Check sheet for the modelled part. Datum: model origin and axes. Units: mm. A direction names the side the tool comes from. Give positions to 0.01 mm unless a question says otherwise; leave off trailing zeros. Loops run counter-clockwise (first coordinate to the right, second up) from the corner with the lowest first, then second, coordinate; pieces in that order, holes last. Notation, with made-up numbers: M 51,-37.75 L 105,-37.75 A25 cw 105,-16.75 Z; hole C 46,58 d8. An arc over 180 degrees is marked long. Put each result on its own line as item: value. Start each with the question number.
```python
from build123d import *

# Parameters (mm, degrees)
BOSS_EXTRUDE1_DEPTH = 3.175
CUT_EXTRUDE1_DEPTH  = 252.960239461
BOSS_EXTRUDE2_DEPTH = 3.175
SKETCH4_R           = 2.159
CUT_EXTRUDE2_DEPTH  = 252.960239461
SKETCH6_W           = 254
SKETCH6_H           = 106.880400145
CUT_EXTRUDE3_DEPTH  = 252.960239461


with BuildPart() as part:
    # Sketch1 → Boss-Extrude1 (new body)
    with BuildSketch(Plane(origin=(0, 0, 0), x_dir=(1, 0, 0), z_dir=(0, 1, 0))):
        Polygon((-152.4, 119.059630377), (-116.478975516, 154.980654861), (116.478975516, 154.980654861), (152.4, 119.059630377), (152.4, -164.698320655), (116.478975516, -200.619345139), (-116.478975516, -200.619345139), (-152.4, -164.698320655), align=None)
    extrude(amount=BOSS_EXTRUDE1_DEPTH)

    # Sketch2 → Cut-Extrude1 (cut, through all)
    with BuildSketch(Plane(origin=(0, 3.175, 0), x_dir=(1, 0, 0), z_dir=(0, 1, 0))):
        Polygon((-91.078975516, 129.580654861), (91.078975516, 129.580654861), (127, 93.659630377), (127, 8.930654861), (82.442975516, 8.930654861), (-74.314975516, 8.930654861), (-127, 8.930654861), (-127, 93.659630377), align=None)
        Polygon((127, -139.298320655), (91.078975516, -175.219345139), (-91.078975516, -175.219345139), (-127, -139.298320655), (-127, -54.569345139), (-74.314975516, -54.569345139), (82.442975516, -54.569345139), (127, -54.569345139), align=None)
    extrude(amount=-CUT_EXTRUDE1_DEPTH, mode=Mode.SUBTRACT)

    # Sketch5 → Boss-Extrude2 (add)
    with BuildSketch(Plane(origin=(0, 3.175, 0), x_dir=(1, 0, 0), z_dir=(0, 1, 0))):
        with BuildLine():
            Line((-116.478975516, 83.138605892), (-80.557951031, 119.059630377))
            ThreePointArc((-80.557951031, 119.059630377), (-78.800891411, 126.352814743), (-72.028975516, 129.580654861))
            Line((-72.028975516, 129.580654861), (-59.328975516, 129.580654861))
            Line((-59.328975516, 129.580654861), (-59.328975516, 154.980654861))
            Line((-59.328975516, 154.980654861), (-116.478975516, 154.980654861))
            Line((-116.478975516, 154.980654861), (-152.4, 119.059630377))
            Line((-152.4, 119.059630377), (-152.4, 65.258187686))
            Line((-152.4, 65.258187686), (-127, 65.258187686))
            Line((-127, 65.258187686), (-127, 77.958187686))
            ThreePointArc((-127, 77.958187686), (-123.351279088, 83.821819005), (-116.478975516, 83.138605892))
        make_face()
        with BuildLine():
            Line((127, 65.258187686), (127, 77.958187686))
            ThreePointArc((127, 77.958187686), (123.351279088, 83.821819005), (116.478975516, 83.138605892))
            Line((116.478975516, 83.138605892), (80.557951031, 119.059630377))
            ThreePointArc((80.557951031, 119.059630377), (78.800891411, 126.352814743), (72.028975516, 129.580654861))
            Line((72.028975516, 129.580654861), (59.328975516, 129.580654861))
            Line((59.328975516, 129.580654861), (59.328975516, 154.980654861))
            Line((59.328975516, 154.980654861), (116.478975516, 154.980654861))
            Line((116.478975516, 154.980654861), (152.4, 119.059630377))
            Line((152.4, 119.059630377), (152.4, 65.258187686))
            Line((152.4, 65.258187686), (127, 65.258187686))
        make_face()
        with BuildLine():
            Line((116.478975516, -128.777296171), (80.557951031, -164.698320655))
            ThreePointArc((80.557951031, -164.698320655), (78.800891411, -171.991505021), (72.028975516, -175.219345139))
            Line((72.028975516, -175.219345139), (59.328975516, -175.219345139))
            Line((59.328975516, -175.219345139), (59.328975516, -200.619345139))
            Line((59.328975516, -200.619345139), (116.478975516, -200.619345139))
            Line((116.478975516, -200.619345139), (152.4, -164.698320655))
            Line((152.4, -164.698320655), (152.4, -110.896877964))
            Line((152.4, -110.896877964), (127, -110.896877964))
            Line((127, -110.896877964), (127, -123.596877964))
            ThreePointArc((127, -123.596877964), (123.351279088, -129.460509283), (116.478975516, -128.777296171))
        make_face()
        with BuildLine():
            Line((-127, -110.896877964), (-127, -123.596877964))
            ThreePointArc((-127, -123.596877964), (-123.351279088, -129.460509283), (-116.478975516, -128.777296171))
            Line((-116.478975516, -128.777296171), (-80.557951031, -164.698320655))
            ThreePointArc((-80.557951031, -164.698320655), (-78.800891411, -171.991505021), (-72.028975516, -175.219345139))
            Line((-72.028975516, -175.219345139), (-59.328975516, -175.219345139))
            Line((-59.328975516, -175.219345139), (-59.328975516, -200.619345139))
            Line((-59.328975516, -200.619345139), (-116.478975516, -200.619345139))
            Line((-116.478975516, -200.619345139), (-152.4, -164.698320655))
            Line((-152.4, -164.698320655), (-152.4, -110.896877964))
            Line((-152.4, -110.896877964), (-127, -110.896877964))
        make_face()
    extrude(amount=-BOSS_EXTRUDE2_DEPTH)

    # Sketch4 → Cut-Extrude2 (cut, through all)
    with BuildSketch(Plane(origin=(0, 3.175, 0), x_dir=(1, 0, 0), z_dir=(0, 1, 0))):
        with Locations(Location((0, 143.550654861, 0), (0, 0, 270))):
            Circle(SKETCH4_R)
        with Locations(Location((-50.8, 143.550654861, 0), (0, 0, 270))):
            Circle(SKETCH4_R)
        with Locations(Location((50.8, 143.550654861, 0), (0, 0, 270))):
            Circle(SKETCH4_R)
        with Locations(Location((-25.4, 143.550654861, 0), (0, 0, 270))):
            Circle(SKETCH4_R)
        with Locations(Location((25.4, 143.550654861, 0), (0, 0, 270))):
            Circle(SKETCH4_R)
        with Locations(Location((-140.97, -22.819345139, 0), (0, 0, 270))):
            Circle(SKETCH4_R)
        with Locations(Location((-140.97, 2.580654861, 0), (0, 0, 270))):
            Circle(SKETCH4_R)
        with Locations(Location((-140.97, 27.980654861, 0), (0, 0, 270))):
            Circle(SKETCH4_R)
        with Locations(Location((140.97, -22.819345139, 0), (0, 0, 270))):
            Circle(SKETCH4_R)
        with Locations(Location((140.97, 2.580654861, 0), (0, 0, 270))):
            Circle(SKETCH4_R)
        with Locations(Location((140.97, 27.980654861, 0), (0, 0, 270))):
            Circle(SKETCH4_R)
        with Locations(Location((140.97, -73.619345139, 0), (0, 0, 90))):
            Circle(SKETCH4_R)
        with Locations(Location((140.97, -48.219345139, 0), (0, 0, 90))):
            Circle(SKETCH4_R)
        with Locations(Location((-140.97, -73.619345139, 0), (0, 0, 90))):
            Circle(SKETCH4_R)
        with Locations(Location((-140.97, -48.219345139, 0), (0, 0, 90))):
            Circle(SKETCH4_R)
        with Locations(Location((25.4, -189.189345139, 0), (0, 0, 90))):
            Circle(SKETCH4_R)
        with Locations(Location((-25.4, -189.189345139, 0), (0, 0, 90))):
            Circle(SKETCH4_R)
        with Locations(Location((50.8, -189.189345139, 0), (0, 0, 90))):
            Circle(SKETCH4_R)
        with Locations(Location((-50.8, -189.189345139, 0), (0, 0, 90))):
            Circle(SKETCH4_R)
        with Locations(Location((0, -189.189345139, 0), (0, 0, 90))):
            Circle(SKETCH4_R)
        with Locations(Location((-76.2, 143.550654861, 0), (0, 0, 270))):
            Circle(SKETCH4_R)
        with Locations(Location((76.2, 143.550654861, 0), (0, 0, 270))):
            Circle(SKETCH4_R)
        with Locations(Location((-140.97, 53.380654861, 0), (0, 0, 270))):
            Circle(SKETCH4_R)
        with Locations(Location((140.97, 53.380654861, 0), (0, 0, 270))):
            Circle(SKETCH4_R)
        with Locations(Location((140.97, -99.019345139, 0), (0, 0, 90))):
            Circle(SKETCH4_R)
        with Locations(Location((76.2, -189.189345139, 0), (0, 0, 90))):
            Circle(SKETCH4_R)
        with Locations(Location((-76.2, -189.189345139, 0), (0, 0, 90))):
            Circle(SKETCH4_R)
        with Locations(Location((-140.97, -99.019345139, 0), (0, 0, 90))):
            Circle(SKETCH4_R)
        with Locations(Location((-140.97, -124.419345139, 0), (0, 0, 270))):
            Circle(SKETCH4_R)
        with Locations(Location((-140.97, 78.780654861, 0), (0, 0, 90))):
            Circle(SKETCH4_R)
        with Locations(Location((140.97, 78.780654861, 0), (0, 0, 270))):
            Circle(SKETCH4_R)
        with Locations(Location((140.97, -124.419345139, 0), (0, 0, 90))):
            Circle(SKETCH4_R)
    extrude(amount=-CUT_EXTRUDE2_DEPTH, mode=Mode.SUBTRACT)

    # Sketch6 → Cut-Extrude3 (cut, through all)
    with BuildSketch(Plane(origin=(0, 3.175, 0), x_dir=(1, 0, 0), z_dir=(0, 1, 0))):
        with Locations((0, -26.175268273)):
            Rectangle(SKETCH6_W, SKETCH6_H)
    extrude(amount=-CUT_EXTRUDE3_DEPTH, mode=Mode.SUBTRACT)


solid = part.part
```
Q1. Section check A-A, the plane z = -13. Record the cut outline in (x, y) (3 decimals), then the cut area to 3 significant figures.
Q2. Depth check by flat-ended pin: P1, Ø3.5, axis at x = 140.97, z = 124.42, coming from the +Y side. Enter the tip coordinate at first touch or a pass-through.
Q3. Section check B-B, the plane x = 95. Record the cut outline in (y, z) (3 decimals).
Q4. Mould release check, pull along Z, two halves, no side actions. Record for faces 3 (the face through (133, 3.175, 20)), 4 (the face through (78.869, 1.61, 171.907)), 5 (the face through (134.7, 1.6, 182.4)): pulls with the +Z half, pulls with the -Z half, needs draft (parallel to the pull), parting line crosses it, or undercut.
Q5. Access from +Z, -Z, +X, -X, +Y, -Y to the whole of each face (thin tool, end or side, straight path). Record for faces 1 (the face through (133, 0, 20)), 2 (the face through (-98.77, 1.61, -100.85)).
Q6. Thickness scan on line 1 along X through (y, z) = (1.55, 122); line 2 along Z through (x, y) = (54.5, 1.5); line 3 along X through (y, z) = (0.5, 129). Record the ranges inside material, lowest first. Write a range as [from, to].
Q7. Section check C-C, the plane y = 2.25. Give the number of separate pieces and of enclosed holes in the cut face, then the cut area to 3 significant figures.
Found:
1. outline: M -152.4,0 L -127,0 L -127,3.175 L -152.4,3.175 Z; M 127,0 L 152.4,0 L 152.4,3.175 L 127,3.175 Z
1. area: 161 mm^2
2. P1: passes through
3. outline: M 0,-154.981 L 3.175,-154.981 L 3.175,-104.618 L 0,-104.618 Z; M 0,150.256 L 3.175,150.256 L 3.175,200.619 L 0,200.619 Z
4. face 3: needs draft
4. face 4: undercut
4. face 5: pulls with the +Z half
5. face 1: +Z, -Z, +X, -X, -Y
5. face 2: +Y, -Y
6. line 1: x = [-152.4, -127], [127, 152.4]
6. line 2: z = [-154.98, -129.58], [175.22, 200.62]
6. line 3: x = [-152.4, -124.14], [-116.79, -116.26], [116.26, 116.79], [124.14, 152.4]
7. separate pieces: 1
7. enclosed holes: 33
7. area: 34,000 mm^2
